Verification items for the finished model (mm, model axes). A direction names the side the tool comes from. Coordinates: 2 decimals unless noted, no trailing zeros. Write each loop counter-clockwise with the first axis right and the second up, starting at its lowest first coordinate (ties: lowest second). Pieces come first, ordered by that corner, then holes. Notation, with made-up numbers: (30.5, 18.25) -> (58.5, 18.25) arc R22 cw to (58.5, 32.25) -> close; hole circle Ø4 at (51, -4). An arc over 180 degrees is marked (long way). Answer in a Markdown table with one row per item.
```python
from build123d import *

# Parameters (mm, degrees)
SKETCH3_R                 = 97.5
BOSS_EXTRUDE3_DEPTH       = 40
SHELL4_T                  = -3
SHELL4_THICKNESS_2_FACE_R = 94.5
SHELL4_THICKNESS_2_DEPTH  = 1.5
CUT_EXTRUDE1_DEPTH        = 2
CUT_EXTRUDE2_REACH        = 145.571
SKETCH5_R                 = 1.5
SKETCH6_R                 = 3.25
CUT_EXTRUDE3_DEPTH        = 0.2
SKETCH7_R                 = 0.48
BOSS_EXTRUDE4_DEPTH       = 1.5
SKETCH8_R                 = 91.5
SKETCH8_R_2               = 90.5
BOSS_EXTRUDE5_DEPTH       = 4
CUT_EXTRUDE12_REACH       = 145.571
SKETCH9_R                 = 2.25
CUT_EXTRUDE13_REACH       = 145.571
SKETCH9_4_W               = 7.5
SKETCH9_4_H               = 22.36


with BuildPart() as part:
    # Sketch3 → Boss-Extrude3 (new body)
    with BuildSketch(Plane(origin=(0, 0, 0), x_dir=(1, 0, 0), z_dir=(0, 1, 0))):
        with Locations(Location((0, 0, 0), (0, 0, 270))):
            Circle(SKETCH3_R)
    extrude(amount=BOSS_EXTRUDE3_DEPTH)

    # Shell4
    shell4_openings = [part.faces().sort_by_distance(p)[0] for p in [
        (0, 40, 0),
    ]]
    offset(amount=SHELL4_T, openings=shell4_openings, kind=Kind.INTERSECTION)

    # Shell4 thickness 2 face (on inner face of the shell) → Shell4 thickness 2 (add)
    with BuildSketch(Plane(origin=(0, 3, 0), x_dir=(0, 0, -1), z_dir=(0, -1, 0))):
        Circle(SHELL4_THICKNESS_2_FACE_R)
    extrude(amount=-SHELL4_THICKNESS_2_DEPTH)

    # Sketch4 → Cut-Extrude1 (cut)
    with BuildSketch(Plane(origin=(0, 4.5, 0), x_dir=(1, 0, 0), z_dir=(0, 1, 0))):
        with BuildLine():
            Line((2.869908719, 1.525163579), (1.543202838, 15.645))
            ThreePointArc((1.543202838, 15.645), (0, 17.05), (-1.543202838, 15.645))
            Line((-1.543202838, 15.645), (-2.869908719, 1.525163579))
            ThreePointArc((-2.869908719, 1.525163579), (-3.25, 0), (-2.869908719, -1.525163579))
            Line((-2.869908719, -1.525163579), (-1.543202838, -15.645))
            ThreePointArc((-1.543202838, -15.645), (0, -17.05), (1.543202838, -15.645))
            Line((1.543202838, -15.645), (2.869908719, -1.525163579))
            ThreePointArc((2.869908719, -1.525163579), (3.25, 0), (2.869908719, 1.525163579))
        make_face()
    extrude(amount=-CUT_EXTRUDE1_DEPTH, mode=Mode.SUBTRACT)

    # Sketch5 → Cut-Extrude2 (cut, up to next)
    with BuildSketch(Plane.XZ, mode=Mode.PRIVATE) as cut_extrude2_sk1:
        with Locations(Location((0, 0, 0), (0, 0, 270))):
            Circle(SKETCH5_R)
    cut_extrude2_tool1 = extrude(cut_extrude2_sk1.sketch, amount=-CUT_EXTRUDE2_REACH, mode=Mode.PRIVATE) & part.part
    add(cut_extrude2_tool1.solids().sort_by_distance((0, 0, 0))[0], mode=Mode.SUBTRACT)

    # Sketch6 → Cut-Extrude3 (cut)
    with BuildSketch(Plane(origin=(0, 2.5, 0), x_dir=(1, 0, 0), z_dir=(0, 1, 0))):
        with Locations(Location((0, 0, 0), (0, 0, 270))):
            Circle(SKETCH6_R)
    extrude(amount=-CUT_EXTRUDE3_DEPTH, mode=Mode.SUBTRACT)

    # Sketch7 → Boss-Extrude4 (add)
    with BuildSketch(Plane(origin=(0, 2.5, 0), x_dir=(1, 0, 0), z_dir=(0, 1, 0))):
        with Locations(Location((0, 15.5, 0), (0, 0, 270))):
            Circle(SKETCH7_R)
        with Locations(Location((0, -15.5, 0), (0, 0, 270))):
            Circle(SKETCH7_R)
    extrude(amount=BOSS_EXTRUDE4_DEPTH)

    # Sketch8 → Boss-Extrude5 (add)
    with BuildSketch(Plane(origin=(0, 4.5, 0), x_dir=(1, 0, 0), z_dir=(0, 1, 0))):
        with Locations(Location((0, 0, 0), (0, 0, 270))):
            Circle(SKETCH8_R)
        with Locations(Location((0, 0, 0), (0, 0, 270))):
            Circle(SKETCH8_R_2, mode=Mode.SUBTRACT)
    extrude(amount=BOSS_EXTRUDE5_DEPTH)

    # Sketch9 → Cut-Extrude12 (cut, up to next)
    with BuildSketch(Plane.XZ, mode=Mode.PRIVATE) as cut_extrude12_sk1:
        with Locations(Location((40.5, 26, 0), (0, 0, 270))):
            Circle(SKETCH9_R)
    cut_extrude12_tool1 = extrude(cut_extrude12_sk1.sketch, amount=-CUT_EXTRUDE12_REACH, mode=Mode.PRIVATE) & part.part
    # Sketch9 → Cut-Extrude12 (cut, up to next)
    with BuildSketch(Plane.XZ, mode=Mode.PRIVATE) as cut_extrude12_sk2:
        with Locations(Location((40.5, 64, 0), (0, 0, 90))):
            Circle(SKETCH9_R)
    cut_extrude12_tool2 = extrude(cut_extrude12_sk2.sketch, amount=-CUT_EXTRUDE12_REACH, mode=Mode.PRIVATE) & part.part
    # Sketch9 → Cut-Extrude12 (cut, up to next)
    with BuildSketch(Plane.XZ, mode=Mode.PRIVATE) as cut_extrude12_sk3:
        with Locations(Location((-40.5, 64, 0), (0, 0, 270))):
            Circle(SKETCH9_R)
    cut_extrude12_tool3 = extrude(cut_extrude12_sk3.sketch, amount=-CUT_EXTRUDE12_REACH, mode=Mode.PRIVATE) & part.part
    # Sketch9 → Cut-Extrude12 (cut, up to next)
    with BuildSketch(Plane.XZ, mode=Mode.PRIVATE) as cut_extrude12_sk4:
        with Locations(Location((-40.5, 26, 0), (0, 0, 90))):
            Circle(SKETCH9_R)
    cut_extrude12_tool4 = extrude(cut_extrude12_sk4.sketch, amount=-CUT_EXTRUDE12_REACH, mode=Mode.PRIVATE) & part.part
    add(cut_extrude12_tool1.solids().sort_by_distance((40.5, 0, 26))[0], mode=Mode.SUBTRACT)
    add(cut_extrude12_tool2.solids().sort_by_distance((40.5, 0, 64))[0], mode=Mode.SUBTRACT)
    add(cut_extrude12_tool3.solids().sort_by_distance((-40.5, 0, 64))[0], mode=Mode.SUBTRACT)
    add(cut_extrude12_tool4.solids().sort_by_distance((-40.5, 0, 26))[0], mode=Mode.SUBTRACT)

    # Sketch9<4> → Cut-Extrude13 (cut, up to next)
    with BuildSketch(Plane.XZ, mode=Mode.PRIVATE) as cut_extrude13_sk1:
        with Locations((40.75, 43.717267505)):
            Rectangle(SKETCH9_4_W, SKETCH9_4_H)
    cut_extrude13_tool1 = extrude(cut_extrude13_sk1.sketch, amount=-CUT_EXTRUDE13_REACH, mode=Mode.PRIVATE) & part.part
    # Sketch9<4> → Cut-Extrude13 (cut, up to next)
    with BuildSketch(Plane.XZ, mode=Mode.PRIVATE) as cut_extrude13_sk2:
        with Locations((-40.75, 43.717267505)):
            Rectangle(SKETCH9_4_W, SKETCH9_4_H)
    cut_extrude13_tool2 = extrude(cut_extrude13_sk2.sketch, amount=-CUT_EXTRUDE13_REACH, mode=Mode.PRIVATE) & part.part
    add(cut_extrude13_tool1.solids().sort_by_distance((40.75, 0, 43.717268))[0], mode=Mode.SUBTRACT)
    add(cut_extrude13_tool2.solids().sort_by_distance((-40.75, 0, 43.717268))[0], mode=Mode.SUBTRACT)


solid = part.part
```
1. Depth check by flat-ended pin: P1, Ø8, axis at x = 70.5, z = -35.5, coming from the -Y side; P2, Ø5, axis at x = 39.5, y = 1.5, coming from the -Z side; P3, Ø1, axis at x = -53, y = 33, coming from the -Z side; P4, Ø3.5, axis at x = 40.5, z = 26, coming from the +Y side. Enter the tip coordinate at first touch or a pass-through.
Geometry says:
| item | result |
|---|---|
| P1 | y = 0 |
| P2 | z = -90.21 |
| P3 | z = -82.16 |
| P4 | through |
2. Section check C-C, the plane x = -40.5. Record the boundary of the cut face in (y, z).
Geometry says:
| item | result |
|---|---|
| outline | (0, -88.69) -> (40, -88.69) -> (40, -85.38) -> (4.5, -85.38) -> (4.5, -82.05) -> (8.5, -82.05) -> (8.5, -80.93) -> (4.5, -80.93) -> (4.5, 23.75) -> (0, 23.75) -> close; (0, 28.25) -> (4.5, 28.25) -> (4.5, 32.54) -> (0, 32.54) -> close; (0, 54.9) -> (4.5, 54.9) -> (4.5, 61.75) -> (0, 61.75) -> close; (0, 66.25) -> (4.5, 66.25) -> (4.5, 80.93) -> (8.5, 80.93) -> (8.5, 82.05) -> (4.5, 82.05) -> (4.5, 85.38) -> (40, 85.38) -> (40, 88.69) -> (0, 88.69) -> close |
3. Section check B-B, the plane y = 33. Record the boundary of the cut face in (x, z).
Geometry says:
| item | result |
|---|---|
| outline | circle Ø195 at (0, 0); hole circle Ø189 at (0, 0) |
4. Tool access check on faces 4 (the cylindrical face through (-92.25, 22, -20.49)), 5 (the flat face through (41, 2, 32.537)). Record the directions out of +Z, -Z, +X, -X, +Y, -Y that give a thin tool (end or side, any length) a straight path to the whole face; none if there is none.
Geometry says:
| item | result |
|---|---|
| face 4 | +Y |
| face 5 | +Y, -Y |
5. Thickness scan on line 1 (X direction, y = 5, z = 0); line 2 (X direction, y = 18, z = 0); line 3 (X direction, y = 2.45, z = 0). Record the ranges inside material, lowest first. Write a range as from..to.
Geometry says:
| item | result |
|---|---|
| line 1 | -97.5..-94.5, -91.5..-90.5, 90.5..91.5, 94.5..97.5 |
| line 2 | -97.5..-94.5, 94.5..97.5 |
| line 3 | -97.5..-3.25, 3.25..97.5 |
6. Section check A-A, the plane z = 64. Record the boundary of the cut face in (x, y), plus the area to 3 significant figures.
Geometry says:
| item | result |
|---|---|
| outline | (-73.55, 0) -> (-42.75, 0) -> (-42.75, 4.5) -> (-63.99, 4.5) -> (-63.99, 8.5) -> (-65.39, 8.5) -> (-65.39, 4.5) -> (-69.53, 4.5) -> (-69.53, 40) -> (-73.55, 40) -> close; (-38.25, 0) -> (38.25, 0) -> (38.25, 4.5) -> (-38.25, 4.5) -> close; (42.75, 0) -> (73.55, 0) -> (73.55, 40) -> (69.53, 40) -> (69.53, 4.5) -> (65.39, 4.5) -> (65.39, 8.5) -> (63.99, 8.5) -> (63.99, 4.5) -> (42.75, 4.5) -> close |
| area | 919 mm^2 |
7. Mould release check, pull along Z, two halves, no side actions. Record for faces 1 (the cylindrical face through (-86.5, 19.72, 44.99)), 2 (the cylindrical face through (42.397, 2.218, 24.79)), 3 (the flat face through (1.4, 0, -1.4)): released by +Z, released by -Z, zero draft, split by the parting line, or undercut.
Geometry says:
| item | result |
|---|---|
| face 1 | split by the parting line |
| face 2 | undercut |
| face 3 | zero draft |
8. Section check D-D, the plane x = 75. Record the boundary of the cut face in (y, z), plus the area to 3 significant figures.
Geometry says:
| item | result |
|---|---|
| outline | (0, -62.3) -> (40, -62.3) -> (40, -57.49) -> (4.5, -57.49) -> (4.5, -52.41) -> (8.5, -52.41) -> (8.5, -50.65) -> (4.5, -50.65) -> (4.5, 50.65) -> (8.5, 50.65) -> (8.5, 52.41) -> (4.5, 52.41) -> (4.5, 57.49) -> (40, 57.49) -> (40, 62.3) -> (0, 62.3) -> close |
| area | 916 mm^2 |
